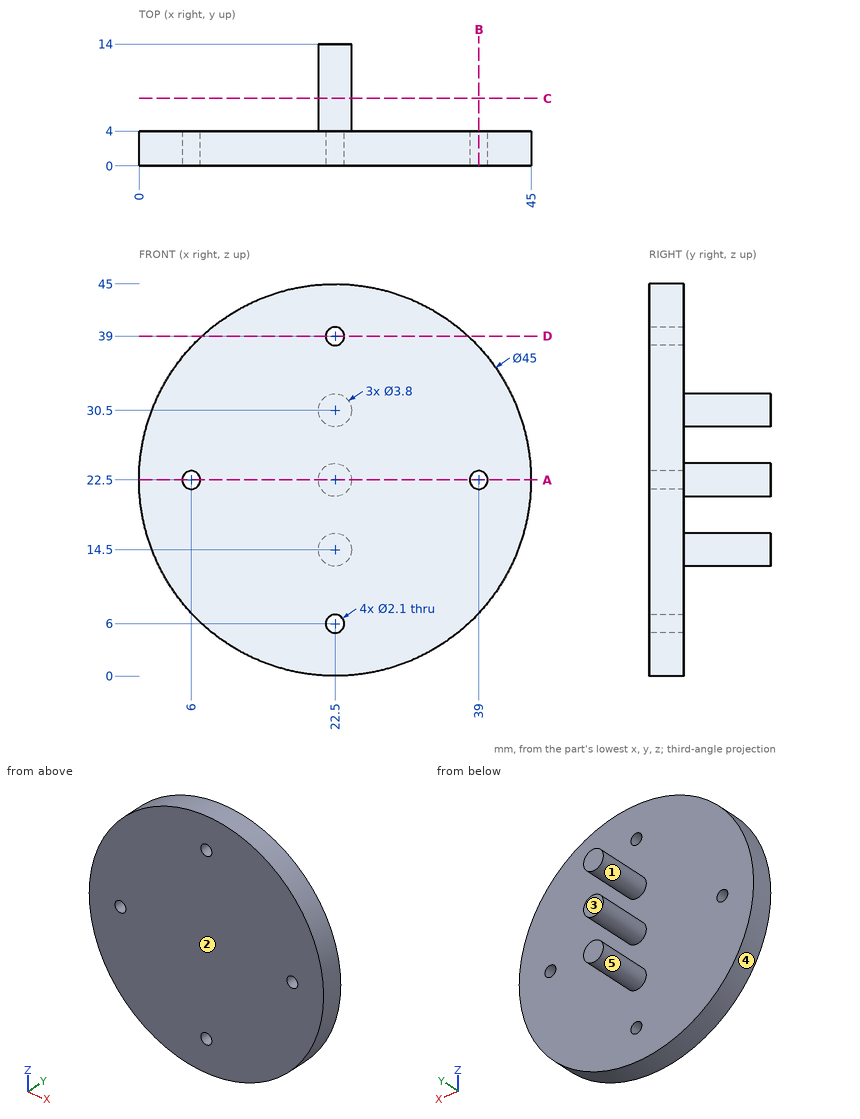
Design review of the part shown in the three views and the two pictorial views. Dimensions are in mm from the part's minimum x, y and z. A direction names the side the tool comes from. Round coordinates to 2 decimals unless told otherwise and drop trailing zeros. Write each loop counter-clockwise with the first axis right and the second up, starting at its lowest first coordinate (ties: lowest second). Pieces come first, ordered by that corner, then holes. Notation, with made-up numbers: (64.25, 78.25) - (96.25, 78.25) arc R25 cw to (96.25, 111.25) - close; hole circle Ø4 at (85.25, 88.5). An arc over 180 degrees is marked (long way). Return JSON: item names as keys, results as strings. Group by question number.
Item 1: Insertion check: P1, Ø1.9, axis at x = 22.5, z = 6, coming from the +Y side; P2, Ø6, axis at x = 7, y = 3, coming from the -Z side; P3, Ø2.5, axis at x = 39, z = 22.5, coming from the +Y side; P4, Ø1, axis at y = 4, z = 31.5, coming from the +X side. Each pin has a flat end and moves straight along its axis. Give the tip position at first contact, or say it passes through.
Item 2: Machinability: for the marked faces 1 and 2, which of the approach directions +Z, -Z, +X, -X, +Y, -Y give a long, thin tool a straight path to every point of the face, cutting with its end or side? Answer none if there is none.
Item 3: We need section B-B on x = 39. Write out the cut boundary in (y, z).
Item 4: For probe 1 along Z at (x, y) = (22.5, 2.7); probe 2 along Z at (x, y) = (23, 9.5); probe 3 along Y at (x, z) = (24.5, 15), list the stretches that pass through material, from the lowest coordinate up. Write a range as [from, to].
Item 5: We need section A-A on z = 22.5. Write out the cut boundary in (x, y), and give its area (3 significant figures).
Item 6: The part is to be moulded in two halves that separate along Z. For the marked faces 3, 4 and 5, say which applies: pulls with the +Z half, pulls with the -Z half, needs draft (parallel to the pull), parting line crosses it, or undercut.
Item 7: We need section D-D on z = 39. Write out the cut boundary in (x, y), and give its area (3 significant figures).
Item 8: We need section C-C on y = 7.75. Write out the cut boundary in (x, z).
Model answer:
{
 "1": {"P1": "passes through", "P2": "stops at z = 3.79", "P3": "stops at y = 4", "P4": "stops at x = 43.33"},
 "2": {"face 1": "+Y", "face 2": "+Z, -Z, +X, -X, -Y"},
 "3": {"outline": "(0, 7.2) - (4, 7.2) - (4, 21.45) - (0, 21.45) - close; (0, 23.55) - (4, 23.55) - (4, 37.8) - (0, 37.8) - close"},
 "4": {"probe 1": "z = [0, 4.95], [7.05, 37.95], [40.05, 45]", "probe 2": "z = [12.67, 16.33], [20.67, 24.33], [28.67, 32.33]", "probe 3": "y = [0, 4]"},
 "5": {"outline": "(0, 0) - (4.95, 0) - (4.95, 4) - (0, 4) - close; (7.05, 0) - (37.95, 0) - (37.95, 4) - (24.4, 4) - (24.4, 14) - (20.6, 14) - (20.6, 4) - (7.05, 4) - close; (40.05, 0) - (45, 0) - (45, 4) - (40.05, 4) - close", "area": "201 mm²"},
 "6": {"face 3": "needs draft", "face 4": "parting line crosses it", "face 5": "undercut"},
 "7": {"outline": "(7.2, 0) - (21.45, 0) - (21.45, 4) - (7.2, 4) - close; (23.55, 0) - (37.8, 0) - (37.8, 4) - (23.55, 4) - close", "area": "114 mm²"},
 "8": {"outline": "circle Ø3.8 at (22.5, 14.5); circle Ø3.8 at (22.5, 22.5); circle Ø3.8 at (22.5, 30.5)"}
}
